The listing builds one solid part. Answer for the finished solid, in the listing's coordinates (mm). A direction names the side the tool comes from. Coordinates: 2 decimals unless noted, no trailing zeros. Write each loop counter-clockwise with the first axis right and the second up, starting at its lowest first coordinate (ties: lowest second). Pieces come first, ordered by that corner, then holes.
from build123d import *
from build123d.topology import SkipClean

# Parameters (mm, degrees)
SKETCH_1_R          = 3.05
EXTRUDE_1_DEPTH     = 2
CUT_EXTRUDE_1_DEPTH = 4.2
FILLET_1_R          = 5


with BuildPart() as part:
    # 草图1 → 凸台-拉伸1 (new, symmetric)
    with BuildSketch(Plane.XY):
        with BuildLine():
            Line((-29, -6), (29, -6))
            ThreePointArc((29, -6), (35, 0), (29, 6))
            Line((29, 6), (-29, 6))
            ThreePointArc((-29, 6), (-35, 0), (-29, -6))
        make_face()
        with Locations((-29, 0)):
            Circle(SKETCH_1_R, mode=Mode.SUBTRACT)
        with Locations((29, 0)):
            Circle(SKETCH_1_R, mode=Mode.SUBTRACT)
    extrude(amount=EXTRUDE_1_DEPTH, both=True)

    # 草图2 → 切除-拉伸1 (cut)
    with SkipClean():  # the faces are left unmerged after this step: merging them gives an invalid solid
        with BuildSketch(Plane.XY.offset(2)):
            with BuildLine():
                Line((23.545643943, -2.5), (-23.545643943, -2.5))
                ThreePointArc((-23.545643943, -2.5), (-25.759629651, -5.049752469), (-29, -6))
                Line((-29, -6), (29, -6))
                ThreePointArc((29, -6), (25.759629651, -5.049752469), (23.545643943, -2.5))
            make_face()
            with BuildLine():
                ThreePointArc((-29, 6), (-25.759629651, 5.049752469), (-23.545643943, 2.5))
                Line((-23.545643943, 2.5), (23.545643943, 2.5))
                ThreePointArc((23.545643943, 2.5), (25.759629651, 5.049752469), (29, 6))
                Line((29, 6), (-29, 6))
            make_face()
        extrude(amount=-CUT_EXTRUDE_1_DEPTH, mode=Mode.SUBTRACT)

    # 圆角1
    fillet_1_edges = [part.edges().sort_by_distance(p)[0] for p in [
        (-23.545643943, -2.5, 0),
        (23.545643943, -2.5, 0),
        (-23.545643943, 2.5, 0),
        (23.545643943, 2.5, 0),
    ]]
    fillet(fillet_1_edges, radius=FILLET_1_R)


solid = part.part
1. Section A-A on y = 0 is taken. Give the vertices of the cut face in (x, z).
Results found:
outline: (-35, -2) - (-32.05, -2) - (-32.05, 2) - (-35, 2) - close; (-25.95, -2) - (25.95, -2) - (25.95, 2) - (-25.95, 2) - close; (32.05, -2) - (35, -2) - (35, 2) - (32.05, 2) - close
2. Section C-C on y = 5 is taken. Give the vertices of the cut face in (x, z), then the cut area to 3 significant figures.
Results found:
outline: (-32.32, -2) - (-25.68, -2) - (-25.68, 2) - (-32.32, 2) - close; (25.68, -2) - (32.32, -2) - (32.32, 2) - (25.68, 2) - close
area: 53.1 mm2
3. Section D-D on x = 15.5 is taken. Give the vertices of the cut face in (y, z), then the cut area to 3 significant figures.
Results found:
outline: (-2.5, -2) - (2.5, -2) - (2.5, 2) - (-2.5, 2) - close
area: 20.0 mm2
4. A tool of negligible diameter and unlimited length cuts with its end or side. For faces 4 (the cylindrical face through (-22.921, -2.904, -0.028)), 5 (the flat face through (0, 0, -2)), 6 (the cylindrical face through (22.974, 2.926, -0.028)), from which of +Z, -Z, +X, -X, +Y, -Y can it reach the whole face along a straight path? Write none if from no direction.
Results found:
face 4: +Z, -Z, -Y
face 5: -Z, +X, -X, +Y, -Y
face 6: +Z, -Z, +Y
5. For a pull along Y with two mould halves and no side action, classify faces 1 (the flat face through (0, 0, 2)), 2 (the cylindrical face through (-26.183, -1.168, -0.028)), 3 (the flat face through (0, 2.5, 0)) as pulls with the +Y half, pulls with the -Y half, needs draft (parallel to the pull), parting line crosses it, or undercut.
Results found:
face 1: needs draft
face 2: undercut
face 3: pulls with the +Y half
6. Section B-B on z = -0.1 is taken. Give the vertices of the cut face in (x, y).
Results found:
outline: (-24.61, -4.09) arc R5 cw to (-20.95, -2.5) - (20.95, -2.5) arc R5 cw to (24.61, -4.09) arc R6 ccw (long way) to (24.61, 4.09) arc R5 cw to (20.95, 2.5) - (-20.95, 2.5) arc R5 cw to (-24.61, 4.09) arc R6 ccw (long way) to start; hole circle Ø6.1 at (-29, 0); hole circle Ø6.1 at (29, 0)
7. Find the intervals of material crossed by L1, parallel to Y at x = -29, z = -0.85; L2, parallel to X at y = 1, z = 1.75; L3, parallel to X at y = -1.5, z = 0.7, in increasing order.
Results found:
L1: y = -6 to -3.05, 3.05 to 6
L2: x = -34.92 to -31.88, -26.12 to 26.12, 31.88 to 34.92
L3: x = -34.81 to -31.66, -26.34 to 26.34, 31.66 to 34.81
8. Flat-ended cylindrical pins translate along their axes: P1, Ø1, axis at x = 16, z = 0.5, coming from the +Y side; P2, Ø7, axis at x = 29, y = 0, coming from the +Z side; P3, Ø2, axis at y = 4.5, z = 1, coming from the -X side; P4, Ø1.2, axis at x = 6, z = 0.5, coming from the -Y side. Find the tip coordinate at first contact, or state that the pin passes through.
Results found:
P1: stops at y = 2.5
P2: stops at z = 2
P3: stops at x = -33.87
P4: stops at y = -2.5
